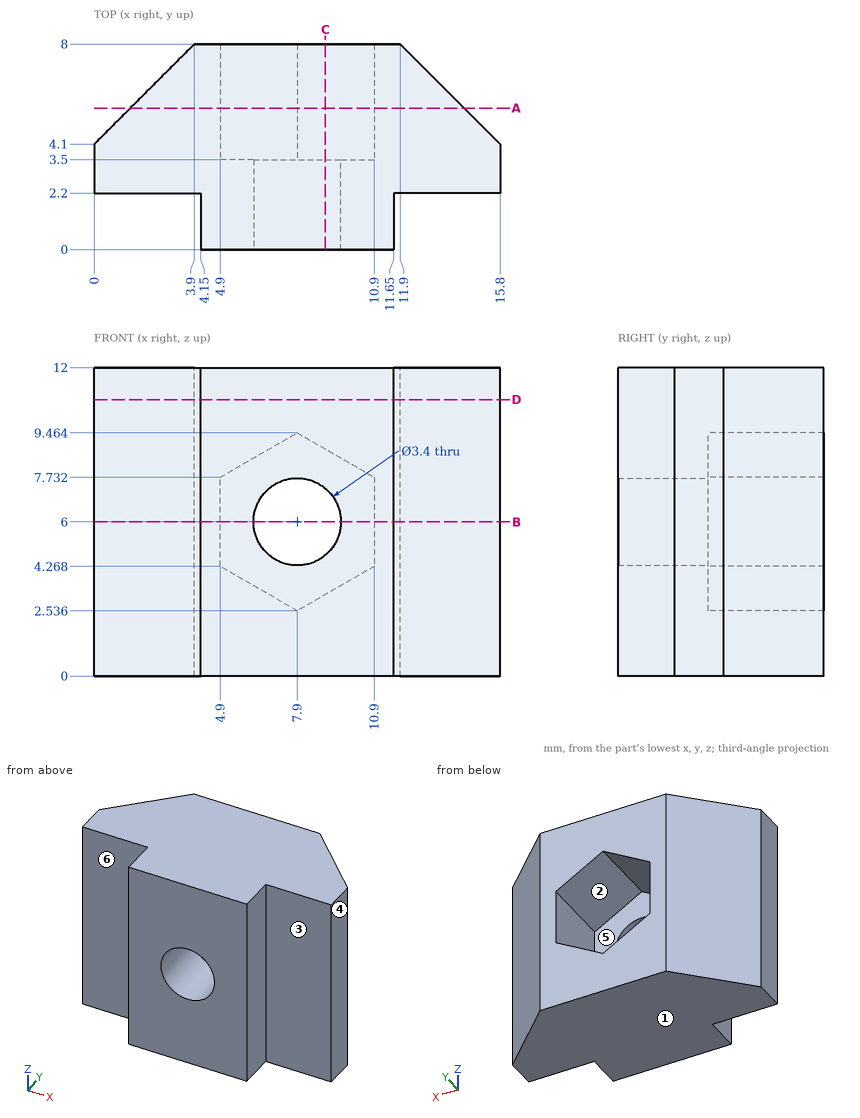
Source: three-view drawing plus pictorial views. Frame: mm from the lowest corner of the part. A direction names the side the tool comes from. Round coordinates to 2 decimals unless told otherwise and drop trailing zeros. Loops run counter-clockwise (first coordinate to the right, second up) from the corner with the lowest first, then second, coordinate; pieces in that order, holes last.
Q1. Material intervals for L1, parallel to Z at x = 7.9, y = 1.85; L2, parallel to Y at x = 6.5, z = 8.5; L3, parallel to X at y = 1.75, z = 3, sorted ascending.
Q2. Pin query (flat end, axial travel): P1, Ø4, axis at x = 7.9, z = 6, coming from the +Y side; P2, Ø1.7, axis at y = 5, z = 5, coming from the +X side; P3, Ø0.7, axis at y = 1, z = 4.5, coming from the -X side. Return the tip coordinate at first contact, or that it passes through.
Q3. Section C-C on x = 9. Return loops of the section in (y, z).
Q4. Section A-A on y = 5.5. Return loops of the section in (x, z).
Q5. Section B-B on z = 6. Return loops of the section in (x, y), plus the area to 3 significant figures.
Q6. Pull-direction query (X, two-part tool) for the marked faces 4, 5 and 6; classes: released by +X, released by -X, zero draft, split by the parting line, or undercut.
Q7. Access query for the marked faces 1, 2 and 3. Directions: +Z, -Z, +X, -X, +Y, -Y. A direction counts if a zero-diameter tool reaches every point of the face in a straight line with its end or side. Return the directions, or none.
Q8. Section D-D on z = 10.75. Return loops of the section in (x, y), plus the area to 3 significant figures.
Evaluation:
1. L1: z = 0 to 4.3, 7.7 to 12
1. L2: y = 0 to 3.5
1. L3: x = 4.15 to 11.65
2. P1: stops at y = 3.5
2. P2: stops at x = 15.75
2. P3: stops at x = 4.15
3. outline: (0, 0) - (8, 0) - (8, 3.17) - (3.5, 3.17) - (3.5, 4.7) - (0, 4.7) - close; (0, 7.3) - (3.5, 7.3) - (3.5, 8.83) - (8, 8.83) - (8, 12) - (0, 12) - close
4. outline: (1.4, 0) - (14.4, 0) - (14.4, 12) - (1.4, 12) - close; hole (4.9, 4.27) - (7.9, 2.54) - (10.9, 4.27) - (10.9, 7.73) - (7.9, 9.46) - (4.9, 7.73) - close
5. outline: (0, 2.2) - (4.15, 2.2) - (4.15, 0) - (6.2, 0) - (6.2, 3.5) - (4.9, 3.5) - (4.9, 8) - (3.9, 8) - (0, 4.1) - close; (9.6, 0) - (11.65, 0) - (11.65, 2.2) - (15.8, 2.2) - (15.8, 4.1) - (11.9, 8) - (10.9, 8) - (10.9, 3.5) - (9.6, 3.5) - close
5. area: 54.0 mm2
6. face 4: released by +X
6. face 5: undercut
6. face 6: zero draft
7. face 1: -Z, +X, -X, +Y, -Y
7. face 2: +Y
7. face 3: +Z, -Z, +X, -Y
8. outline: (0, 2.2) - (4.15, 2.2) - (4.15, 0) - (11.65, 0) - (11.65, 2.2) - (15.8, 2.2) - (15.8, 4.1) - (11.9, 8) - (3.9, 8) - (0, 4.1) - close
8. area: 92.9 mm2
